Check sheet for the modelled part. Datum: model origin and axes. Units: mm. Face numbers are marked on the shaded views. A direction names the side the tool comes from. Round coordinates to 2 decimals unless told otherwise and drop trailing zeros. Order: outer loops, then holes, each group sorted by start corner. A loop starts at its lowest first (then second) coordinate and runs counter-clockwise, first axis right, second up. Notation, with made-up numbers: (27.5, 40.5) -> (34.5, 40.5) arc R16 ccw to (34.5, 70.5) -> close; hole circle Ø10 at (48.25, -1). An arc over 180 degrees is marked (long way). Answer in a Markdown table with one row per item. Add a question column.
1. Draft check along Z on the marked faces 3, 4 and 5. Enter one of: +Z half, -Z half, draft (parallel to the pull), parting line (faces both ways), or undercut.
2. Material ranges on L1, parallel to Y at x = 0, z = -6.7; L2, parallel to Y at x = 0, z = -10.2; L3, parallel to Z at x = -4.5, y = -2, recorded low to high. Write a range as from..to.
3. Sectioned sample at A-A, the plane y = 0. Record the boundary of the cut face in (x, z), then the cut area to 3 significant figures.
4. Sectioned sample at C-C, the plane z = -3. Record the boundary of the cut face in (x, y).
5. Access from +Z, -Z, +X, -X, +Y, -Y to the whole of each face (thin tool, end or side, straight path). Record for the marked faces 1 and 2.
6. Depth check by flat-ended pin: P1, Ø6.5, axis at x = -1, y = -1.5, coming from the -Z side; P2, Ø14.5, axis at x = -2.5, y = 0, coming from the -Z side; P3, Ø2, axis at x = 5, z = -7.5, coming from the +Y side; P4, Ø1.5, axis at x = 14.5, y = -11, coming from the -Z side. Enter the tip coordinate at first touch or a pass-through.
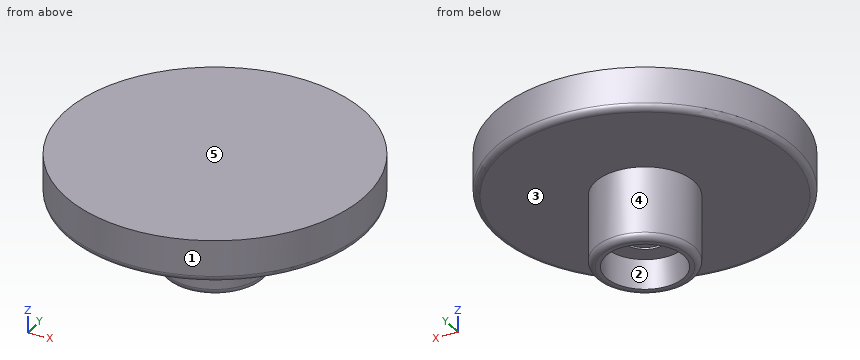
Autodesk Fusion 360 part; units mm, degrees
sketch "Sketch1" plane through (0, 0, 0) normal (0, 0, 1) x (1, 0, 0)
  circle A0 centre (0, 0) radius 8.25
  circle A1 centre (0, 0) radius 6.5
  circle A2 centre (0, 0) radius 3.05
  circle A3 centre (0, 0) radius 3.55
  circle A4 centre (0, 0) radius 25
  dimension "d1" = 16.5
  dimension "d2" = 13
  dimension "d7" = 6.1
  dimension "d8" = 7.1
  dimension "d9" = 50
extrude "Extrude1" add sketch "Sketch1" against normal blind 12 contours A0
extrude "Extrude2" add sketch "Sketch1" against normal blind 7 contours A1 | A2 | A3
extrude "Extrude3" add sketch "Sketch1" against normal blind 8 contours A3
extrude "Extrude4" cut 1 faces at (3.3701, -0.1764, -8) along direction (0, 0, 1) blind 1.5
extrude "Extrude5" add sketch "Sketch1" along normal blind 7 contours A0 | A1 | A2 | A3 | A4
fillet "Fillet1" radius 1 2 edges at (-7.6917, 2.9833, -12) (-23.3082, -9.0404, 0)
Answer key:
| question | item | result |
|---|---|---|
| 1 | face 3 | -Z half |
| 1 | face 4 | draft |
| 1 | face 5 | +Z half |
| 2 | L1 | y = -8.25..-3.55, -3.05..3.05, 3.55..8.25 |
| 2 | L2 | y = -8.25..-6.5, 6.5..8.25 |
| 2 | L3 | z = -7..7 |
| 3 | outline | (-25, 1) arc R1 ccw to (-24, 0) -> (-8.25, 0) -> (-8.25, -11) arc R1 ccw to (-7.25, -12) -> (-6.5, -12) -> (-6.5, -7) -> (-3.55, -7) -> (-3.55, -6.5) -> (-3.05, -6.5) -> (-3.05, -7) -> (3.05, -7) -> (3.05, -6.5) -> (3.55, -6.5) -> (3.55, -7) -> (6.5, -7) -> (6.5, -12) -> (7.25, -12) arc R1 ccw to (8.25, -11) -> (8.25, 0) -> (24, 0) arc R1 ccw to (25, 1) -> (25, 7) -> (-25, 7) -> close |
| 3 | area | 482 mm² |
| 4 | outline | circle Ø16.5 at (0, 0) |
| 5 | face 1 | +Z, -Z |
| 5 | face 2 | -Z |
| 6 | P1 | stops at z = -7 |
| 6 | P2 | stops at z = -12 |
| 6 | P3 | stops at y = 7.22 |
| 6 | P4 | stops at z = 0 |
